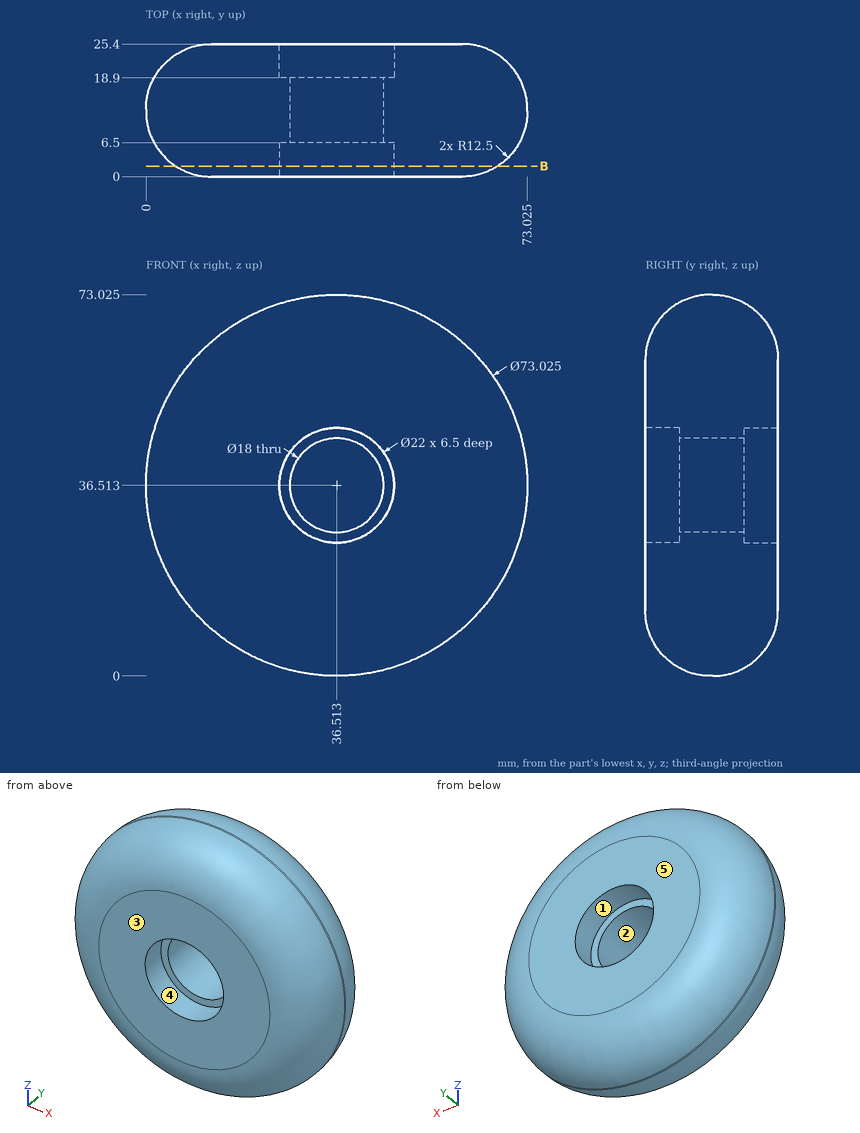
Could you check a few things on this drawing? It's one solid part, dimensions in mm from its lowest x, y, z. A direction names the side the tool comes from. Coordinates: 2 decimals unless noted, no trailing zeros. Order: outer loops, then holes, each group sorted by start corner. A loop starts at its lowest first (then second) coordinate and runs counter-clockwise, first axis right, second up. Notation, with made-up numbers: M 73,35 L 103,35 A17 cw 103,66 Z; hole C 35.5,19.5 d11. An arc over 180 degrees is marked long. Use a Markdown table: item, result. Add a question column.
Q1. I want a section at B-B on y = 2. List the corners of the cut face in (x, z) for me (1 decimal), then the cut area to 3 significant figures.
Q2. Which directions (+Z, -Z, +X, -X, +Y, -Y) give clear straight access to the entire face, cutting with the end or side of a thin tool? Please do the marked faces 4 and 5.
Q3. I'm going to push flat-ended pins straight in: pin 1 (12 mm diameter, centred on x = 15.5, y = 6, fed in from +Z); pin 2 (17.5 mm diameter, centred on x = 36.51, z = 36.51, fed in from +Y); pin 3 (2 mm diameter, centred on y = 7.5, z = 63.5, fed in from -X) (1 decimal); pin 4 (1 mm diameter, centred on x = 61.5, z = 60.5, fed in from -Y). Where does each tip first touch, or does it pass through?
Q4. We'd pull the mould along X, two halves only. Please class the marked faces 1, 2 and 3: pulls with the +X half, pulls with the -X half, needs draft (parallel to the pull), parting line crosses it, or undercut.
Q5. If I drill on L1, parallel to X at y = 3.75, z = 26.5 (1 decimal); L2, parallel to Z at x = 40.5, y = 14.5 (1 decimal); L3, parallel to Z at x = 41, y = 23 (1 decimal), over which ranges is the centre line in solid material (lowest first)?
Checked values:
| question | item | result |
|---|---|---|
| 1 | outline | C 36.5,36.5 d61.6; hole C 36.5,36.5 d22 |
| 1 | area | 2,600 mm² |
| 2 | face 4 | -Y |
| 2 | face 5 | +Z, -Z, +X, -X, +Y |
| 3 | pin 1 | z = 68.87 |
| 3 | pin 2 | through |
| 3 | pin 3 | x = 12.2 |
| 3 | pin 4 | y = 5.17 |
| 4 | face 1 | undercut |
| 4 | face 2 | undercut |
| 4 | face 3 | needs draft |
| 5 | L1 | 5.1 to 32, 41.1 to 67.9 |
| 5 | L2 | 0.3 to 28.4, 44.6 to 72.7 |
| 5 | L3 | 5.5 to 26.5, 46.6 to 67.6 |
